Geometry: final body of the model. Coordinates: model frame, mm. A direction names the side the tool comes from. Round coordinates to 2 decimals unless told otherwise and drop trailing zeros. Loops run counter-clockwise (first coordinate to the right, second up) from the corner with the lowest first, then second, coordinate; pieces in that order, holes last. Notation, with made-up numbers: (51.5, -40) - (73.5, -40) arc R22 cw to (73.5, -24) - close; hole circle Ø3 at (59.25, -19.75). An arc over 180 degrees is marked (long way). Answer as a JSON object with one key per item and string values. Group by question number.
Item 1: Section D-D (x = 3.75). Return the cut outline in (y, z), plus the area to 3 significant figures.
Item 2: Section C-C (y = 2.5). Return the cut outline in (x, z).
Item 3: Section A-A (y = 17.75). Return the cut outline in (x, z).
Item 4: Reachability of faces 1 (the face through (0, 12, 3)), 2 (the face through (-1.034, 17.506, 1.479)) from +Z, -Z, +X, -X, +Y, -Y: full face, straight path, thin tool, end or side. Return the list, or none.
Item 5: First-contact query: pin 1 (10 mm diameter, centred on y = 9.5, z = 6.5, fed in from +X); pin 2 (2 mm diameter, centred on x = 7.5, z = 6.5, fed in from +Y); pin 3 (7 mm diameter, centred on x = 1.5, y = 15, fed in from +Z). Flat tips, straight axial feed; report the tip coordinate or a pass-through.
Item 6: Section B-B (z = 28.5). Return the cut outline in (x, y), plus the area to 3 significant figures.
Item 7: Draft query along Z for faces 3 (the face through (0, 10, 0)), 4 (the face through (-3, 3, 11)), 5 (the face through (-2.703, 1.479, 11.416)). Return one class per face: released by +Z, released by -Z, zero draft, split by the parting line, or undercut.
Item 8: Line query: line 1 (X direction, y = 2.25, z = 20); line 2 (Z direction, x = 0, y = 0.75); line 3 (Z direction, x = -7, y = 4.5). Output: solid intervals per line, ascending.
```python
from build123d import *

# Parameters (mm, degrees)
PAD_DEPTH    = 3
PAD001_DEPTH = 3


with BuildPart() as part:
    # Sketch → Pad (new body)
    with BuildSketch(Plane.XY):
        with BuildLine():
            ThreePointArc((0, 17.3), (2.7, 20), (0, 22.7))
            Line((0, 25.7), (0, 22.7))
            ThreePointArc((5.344781, 21.980735), (3.255749, 24.678685), (0, 25.7))
            Line((11.644779, 4.980742), (5.344781, 21.980735))
            ThreePointArc((12, 3), (11.910492, 4.006171), (11.644779, 4.980742))
            Line((12, 0), (12, 3))
            Line((0, 0), (12, 0))
            Line((0, 17.3), (0, 0))
        make_face()
    pad = extrude(amount=PAD_DEPTH)

    # Sketch001 → Pad001 (join)
    with BuildSketch(Plane.XZ):
        with BuildLine():
            ThreePointArc((0, 11), (9, 20), (0, 29))
            Line((0, 29), (0, 32))
            ThreePointArc((12, 20.000045), (8.485265, 28.485297), (0, 32))
            Line((12, 20.000045), (12, 3))
            Line((12, 3), (12, 0))
            Line((12, 0), (0, 0))
            Line((0, 0), (0, 11))
        make_face()
    pad001 = extrude(amount=-PAD001_DEPTH)

    # Mirrored: Pad, Pad001 across Sketch V_Axis
    add(pad.mirror(Plane(origin=(0, 0, 0), x_dir=(0, 0, 1), z_dir=(1, 0, 0))))
    add(pad001.mirror(Plane(origin=(0, 0, 0), x_dir=(0, 0, 1), z_dir=(1, 0, 0))))


solid = part.part
```
Values:
{
 "1": {"outline": "(0, 0) - (24.29, 0) - (24.29, 3) - (3, 3) - (3, 11.82) - (0, 11.82) - close; (0, 28.18) - (3, 28.18) - (3, 31.4) - (0, 31.4) - close", "area": "109 mm^2"},
 "2": {"outline": "(-12, 0) - (12, 0) - (12, 20) arc R12 ccw to (0, 32) arc R12 ccw to (-12, 20) - close; hole circle Ø18 at (0, 20)"},
 "3": {"outline": "(-6.91, 0) - (-1.49, 0) - (-1.49, 3) - (-6.91, 3) - close; (1.49, 0) - (6.91, 0) - (6.91, 3) - (1.49, 3) - close"},
 "4": {"face 1": "+Z, +X, -X, +Y", "face 2": "+Z, -Z"},
 "5": {"pin 1": "stops at x = 11.29", "pin 2": "stops at y = 3", "pin 3": "stops at z = 3"},
 "6": {"outline": "(-8.47, 0) - (-2.96, 0) - (-2.96, 3) - (-8.47, 3) - close; (2.96, 0) - (8.47, 0) - (8.47, 3) - (2.96, 3) - close", "area": "33.1 mm^2"},
 "7": {"face 3": "released by -Z", "face 4": "zero draft", "face 5": "undercut"},
 "8": {"line 1": "x = -12 to -9, 9 to 12", "line 2": "z = 0 to 11, 29 to 32", "line 3": "z = 0 to 3"}
}
